Autodesk Inventor part; units mm, degrees
ref_plane "YZ Plane" through (0, 0, 0) normal (1, 0, 0) x (0, 1, 0)
ref_plane "XZ Plane" through (0, 0, 0) normal (0, 1, 0) x (-1, 0, 0)
ref_plane "XY Plane" through (0, 0, 0) normal (0, 0, 1) x (1, 0, 0)
sketch "Sketch1" plane through (0, 0, 0) normal (0, 0, 1) x (1, 0, 0)
  line L0 (-74.9186, 47.1822) -> (53.4099, 57.2393) construction
  line L1 (53.4099, 57.2393) -> (63.1167, -66.6187) construction
  line L2 (63.1167, -66.6187) -> (-65.2118, -76.6758) construction
  line L3 (-65.2118, -76.6758) -> (-74.9186, 47.1822) construction
  line L4 (6, 16) -> (-6, 24) construction
  line L5 (0, 20) -> (6, 24) construction
  circle A0 centre (1.0672, -0.4938) radius 75
  line L6 (1.0672, 74.5062) -> (1.0672, -0.4938) construction
  line L7 (1.0672, 74.5062) -> (5.6579, 61.8933)
  line L8 (1.0672, 74.5062) -> (14.4896, 74.5062) construction
  line L9 (1.3501, 55.1985) -> (-17.016, 53.7591)
  line L10 (-17.016, 53.7591) -> (-67, 31)
  arc A1 (1.3501, 55.1985) -> (5.6579, 61.8933) centre (0.9595, 60.1832) ccw
  circle A2 centre (1.0672, -0.4938) radius 20
  point P0 (0, 0)
  point P1 (7.9076, 55.7124)
  dimension "d2" = 12
  dimension "d4" = 150
  dimension "d5" = 20
  dimension "d6" = 70
  dimension "d8" = 25
  dimension "d10" = 160
  dimension "d11" = 5
  dimension "d23" = 40
ref_plane "Work Plane1" through (0, 0, 0) normal (0, 0, -1) x (-1, 0, 0)
sketch "Sketch2" plane through (0, 0, 0) normal (0, 0, -1) x (-1, 0, 0)
  line L0 (0, 75) -> (-4.3981, 62.9162)
  arc A0 (-4.3981, 62.9162) -> (0.3003, 56.2061) centre (0.3003, 61.2061) ccw
  line L1 (0.3003, 56.2061) -> (18.1596, 56.2061)
  line L2 (18.1596, 56.2061) -> (63.6666, 39.643)
  arc A1 (63.6666, 39.643) -> (0, 75) centre (27.2068, 48.9906) ccw
  point P0 (0, 0)
extrude "Extrusion3" add sketch "Sketch1" along normal blind 15
extrude "Extrusion4" cut sketch "Sketch2" against normal blind 15
pattern_circular "Circular Pattern2" count 3 over 360 about axis through (1.0672, -0.4938, 0) along (0, 0, 1) of "Extrusion4"
sketch "Sketch3" plane through (0, 0, 0) normal (0, 0, -1) x (-1, 0, 0)
  circle A0 centre (-1.0672, -0.4938) radius 20
  point P0 (0, 0)
sketch "Sketch4" plane through (0, 0, 15) normal (0, 0, 1) x (1, 0, 0)
  circle A0 centre (1.0672, -0.4938) radius 20
  line L0 (17.9236, 2.3101) -> (11.9236, 12.7024)
  line L1 (11.9236, 12.7024) -> (18.8518, 16.7024)
  line L2 (18.8518, 16.7024) -> (24.8518, 6.3101)
  line L3 (24.8518, 6.3101) -> (17.9236, 2.3101)
  line L4 (17.9236, 2.3101) -> (18.8518, 16.7024) construction
  line L5 (11.9236, 12.7024) -> (24.8518, 6.3101) construction
  point P0 (0, 0)
  point P1 (18.3877, 9.5062)
  dimension "d35" = 12
  dimension "d36" = 8
extrude "Extrusion5" cut sketch "Sketch4" against normal through all contours L3 L0 L1 A0 | A0 L1 L2 L3 picked at (15.7106, 8.7411)
properties part number "pisau ok2" material "Stainless Steel"
Can you work these out from the model? Positions are in its coordinate system, mm. A direction names the side the tool comes from. Round coordinates to 2 decimals unless told otherwise and drop trailing zeros. Write each loop counter-clockwise with the first axis right and the second up, starting at its lowest first coordinate (ties: lowest second). Pieces come first, ordered by that corner, then holes. Notation, with made-up numbers: M 51,27.5 L 97,27.5 A32 cw 97,53.5 Z; hole C 53,-26 d5. An arc over 180 degrees is marked long. Use CSV: the item, a comma, the result in double quotes.
(1) On a 3-axis mill with a long thin cutter (end or side, diameter ignored), from which of +Z, -Z, +X, -X, +Y, -Y can I reach the whole of each face in a straight line? I mean faces 4 (the flat face through (-59.53, -34.1, 7.4)), 5 (the flat face through (21.81, 11.58, 7.6)), 6 (the flat face through (55.26, -20.03, 7.4)). Say none if no direction works.
Check values:
face 4,"+Z, -Z, -Y"
face 5,"+Z, -Z"
face 6,"+Z, -Z, +X"
(2) Imagine slicing it at A-A (z = 9.25). Write out the boundary of the cut face in (x, y).
Check values:
outline,"M -63.44,-38.76 L -55.51,-29.31 A5 cw -47.35,-30.03 L -38.42,-45.49 L -2.79,-75.39 A75 ccw 66.46,-37.22 L 54.32,-35.08 A5 cw 50.85,-27.66 L 59.78,-12.19 L 67.86,33.62 A75 ccw 0.18,74.5 L 4.4,62.92 A5 cw -0.3,56.21 L -18.16,56.21 L -61.87,40.3 A75 ccw Z; hole M 14.59,14.24 A20 ccw long 20.59,3.85 L 24.85,6.31 L 18.85,16.7 Z"
(3) I need wall thicknesses on line 1 along X through (y, z) = (16, 9.25); line 2 along Y through (x, z) = (-15.5, 13.75); line 3 along X through (y, z) = (-16, 9). Which ranges of each line are inside material? Lowest first, please.
Check values:
line 1,"-72.1 to -10.24, 12.38 to 17.64, 19.26 to 64.76"
line 2,"-64.73 to -11.7, 10.71 to 56.21"
line 3,"-72.31 to -11.56, 13.7 to 57.59"
(4) Imagine slicing it at C-C (y = 29.5). Write out the boundary of the cut face in (x, z).
Check values:
outline,"M -67.67,0 L 67.14,0 L 67.14,15 L -67.67,15 Z"
(5) I'm going to push flat-ended pins straight in: pin 1 (7.5 mm diameter, centred on x = -6.5, z = 6, fed in from +Y); pin 2 (5 mm diameter, centred on x = -58, z = 13, fed in from -Y); pin 3 (5 mm diameter, centred on y = -59, z = 8.5, fed in from -X). Where does each tip first touch, or does it pass through?
Check values:
pin 1,"y = 56.21"
pin 2,"y = -35.26"
pin 3,"x = -25.31"
(6) We'd pull the mould along X, two halves only. Please class faces 1 (the flat face through (16.691, 15.455, 7.605)), 2 (the flat face through (60.47, -36.17, 7.4)), 3 (the flat face through (-20.9, -60.2, 7.4)): +X half, -X half, draft (parallel to the pull), parting line (faces both ways), or undercut.
Check values:
face 1,"undercut"
face 2,"+X half"
face 3,"-X half"
(7) Imagine slicing it at D-D (x = -52). Write out the boundary of the cut face in (y, z).
Check values:
outline,"M -27.54,0 L 43.89,0 L 43.89,15 L -27.54,15 Z"
(8) Imagine slicing it at B-B (x = 2.5). Write out the boundary of the cut face in (y, z), plus the area to 3 significant figures.
Check values:
outline,"M -75.48,0 L -20.44,0 L -20.44,15 L -75.48,15 Z; M 19.45,0 L 57.06,0 L 57.06,15 L 19.45,15 Z; M 68.13,0 L 74.49,0 L 74.49,15 L 68.13,15 Z"
area,"1,490 mm^2"
